Input: part model. Units: mm. Frame: model coordinates. A direction names the side the tool comes from. Coordinates: 2 decimals unless noted, no trailing zeros. Order: outer loops, then holes, each group sorted by start corner. A loop starts at its lowest first (then second) coordinate and runs counter-clockwise, first axis right, second up. Notation, with made-up numbers: (-1.5, -3.5) -> (12.5, -3.5) arc R20 cw to (12.5, 20.5) -> close; hole circle Ø5 at (31, 37). An arc over 180 degrees is marked (long way). One line per question, with ' | ' between items.
```python
from build123d import *

# Parameters (mm, degrees)
SKETCH1_W           = 38
SKETCH1_H           = 44
BOSS_EXTRUDE1_DEPTH = 27.5
SKETCH2_W           = 20
SKETCH2_H           = 16
CUT_EXTRUDE1_DEPTH  = 55
SKETCH3_R           = 14
CUT_EXTRUDE2_DEPTH  = 55
SKETCH4_W           = 7
SKETCH4_H           = 28
CUT_EXTRUDE3_DEPTH  = 65.313684391


with BuildPart() as part:
    # Sketch1 → Boss-Extrude1 (new, symmetric)
    with BuildSketch(Plane.XY):
        with Locations((19, 22)):
            Rectangle(SKETCH1_W, SKETCH1_H)
    extrude(amount=BOSS_EXTRUDE1_DEPTH, both=True)

    # Sketch2 → Cut-Extrude1 (cut)
    with BuildSketch(Plane.XY.offset(27.5)):
        with Locations((19, 22)):
            Rectangle(SKETCH2_W, SKETCH2_H)
    extrude(amount=-CUT_EXTRUDE1_DEPTH, mode=Mode.SUBTRACT)

    # Sketch3 → Cut-Extrude2 (cut)
    with BuildSketch(Plane(origin=(38, 0, 0), x_dir=(0, 0, -1), z_dir=(1, 0, 0))):
        with Locations((-3.5, 22)):
            Circle(SKETCH3_R)
    extrude(amount=-CUT_EXTRUDE2_DEPTH, mode=Mode.SUBTRACT)

    # Sketch4 → Cut-Extrude3 (cut, through all)
    with BuildSketch(Plane(origin=(38, 0, 0), x_dir=(0, 0, -1), z_dir=(1, 0, 0))):
        with Locations((24, 22)):
            Rectangle(SKETCH4_W, SKETCH4_H)
    extrude(amount=-CUT_EXTRUDE3_DEPTH, mode=Mode.SUBTRACT)


solid = part.part
```
1. Access query for faces 4 (the face through (9, 22, -16)), 5 (the face through (19, 36, -24)), 6 (the face through (19, 40, -27.5)). Directions: +Z, -Z, +X, -X, +Y, -Y. A direction counts if a zero-diameter tool reaches every point of the face in a straight line with its end or side. Return the directions, or none.
Recorded:
face 4: +Z, -Z | face 5: -Z, +X, -X | face 6: -Z, +X, -X, +Y, -Y
2. Ray query, line 1 (Y direction, x = 16.5, z = -18); line 2 (Y direction, x = 9, z = -24); line 3 (X direction, y = 16, z = 16.5). Return the intervals inside material, ascending. Write a range as [from, to].
Recorded:
line 1: y = [0, 14], [30, 44] | line 2: y = [0, 8], [36, 44] | line 3: x = [0, 9], [29, 38]
3. Cut plane A-A, the plane x = 33. Return loops of the section in (y, z).
Recorded:
outline: (0, -27.5) -> (8, -27.5) -> (8, -20.5) -> (36, -20.5) -> (36, -27.5) -> (44, -27.5) -> (44, 27.5) -> (0, 27.5) -> close; hole circle Ø28 at (22, 3.5)
4. Cut plane B-B, the plane y = 22. Return loops of the section in (x, z).
Recorded:
outline: (0, -20.5) -> (9, -20.5) -> (9, -10.5) -> (0, -10.5) -> close; (0, 17.5) -> (9, 17.5) -> (9, 27.5) -> (0, 27.5) -> close; (29, -20.5) -> (38, -20.5) -> (38, -10.5) -> (29, -10.5) -> close; (29, 17.5) -> (38, 17.5) -> (38, 27.5) -> (29, 27.5) -> close
5. Cut plane D-D, the plane x = 12.5. Return loops of the section in (y, z).
Recorded:
outline: (0, -27.5) -> (8, -27.5) -> (8, -20.5) -> (14, -20.5) -> (14, -7.99) arc R14 cw to (14, 14.99) -> (14, 27.5) -> (0, 27.5) -> close; (30, -20.5) -> (36, -20.5) -> (36, -27.5) -> (44, -27.5) -> (44, 27.5) -> (30, 27.5) -> (30, 14.99) arc R14 cw to (30, -7.99) -> close
6. Cut plane C-C, the plane z = -19.5. Return loops of the section in (x, y), and give its area (3 significant figures).
Recorded:
outline: (0, 0) -> (38, 0) -> (38, 44) -> (0, 44) -> close; hole (9, 14) -> (29, 14) -> (29, 30) -> (9, 30) -> close | area: 1,350 mm^2
7. Pin query (flat end, axial travel): pin 1 Ø22.5 at (x, y) = (13.5, 21) entering from -Z; pin 2 Ø8 at (x, y) = (25.5, 29.5) entering from +Z. Return the tip coordinate at first contact, or that it passes through.
Recorded:
pin 1: stops at z = -20.5 | pin 2: stops at z = 27.5
8. Mould query, pull axis Y, two halves, no side actions, for faces 1 (the face through (19, 8, -24)), 2 (the face through (19, 32, 27.5)), 3 (the face through (19, 44, 0)). Classes: released by +Y, released by -Y, zero draft, split by the parting line, or undercut.
Recorded:
face 1: undercut | face 2: zero draft | face 3: released by +Y
